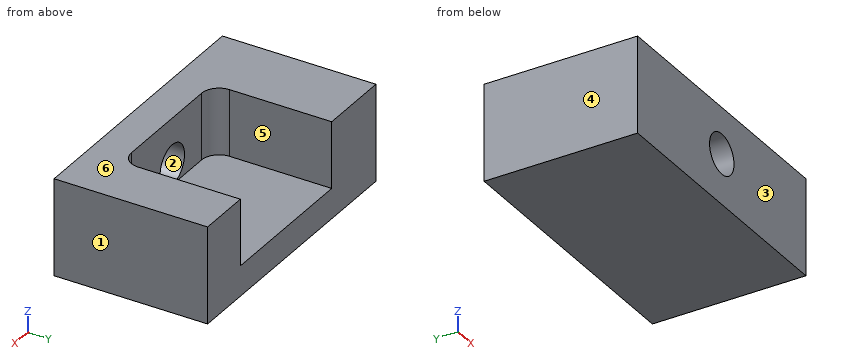
```python
from build123d import *

# Parameters (mm, degrees)
F0_W     = 56.4152672887
F0_H     = 35.5571135879
F1_DEPTH = 101.6
F3_DEPTH = 24.4419761002
F4_R     = 7.3661777125
F5_DEPTH = 25.4


with BuildPart() as f1:
    # F0 (on Right) → F1 (new body)
    with BuildSketch(Plane.YZ):
        with Locations((28.2076336443, 17.7785567939)):
            Rectangle(F0_W, F0_H)
    extrude(amount=F1_DEPTH)

    # F2 (on face) → F3 (cut)
    with BuildSketch(Plane.XY.offset(35.5571135879)):
        with BuildLine():
            Line((81.8312615156, 18.8686089426), (81.8312615156, 56.4152672887))
            Line((81.8312615156, 56.4152672887), (26.6845934093, 56.4152672887))
            Line((26.6845934093, 56.4152672887), (26.6845934093, 18.8686089426))
            ThreePointArc((26.6845934093, 18.8686089426), (28.5444653488, 14.3784808821), (33.0345934093, 12.5186089426))
            Line((33.0345934093, 12.5186089426), (75.4812615156, 12.5186089426))
            ThreePointArc((75.4812615156, 12.5186089426), (79.9713895762, 14.3784808821), (81.8312615156, 18.8686089426))
        make_face()
    extrude(amount=-F3_DEPTH, mode=Mode.SUBTRACT)

    # F4 (on face) → F5 (cut)
    with BuildSketch(Plane.XZ):
        with Locations((50.8, 18.4632241726)):
            Circle(F4_R)
    extrude(amount=-F5_DEPTH, mode=Mode.SUBTRACT)


solid = f1.part
```
Source: CAD feature listing. Evaluate the final solid. Frame: model axes, mm. Face numbers are marked on the shaded views. A direction names the side the tool comes from. Give positions to 0.01 mm unless a question says otherwise; leave off trailing zeros. Loops run counter-clockwise (first coordinate to the right, second up) from the corner with the lowest first, then second, coordinate; pieces in that order, holes last. Notation, with made-up numbers: (85.25, 27) - (103.25, 27) arc R17 ccw to (103.25, 32) - close; hole circle Ø9 at (49, 84.25). An arc over 180 degrees is marked (long way). Use CSV: the item, a comma, the result in double quotes. Start each with the question number.
1. Draft query along X for the marked faces 1, 2, 3 and 4. Return one class per face: +X half, -X half, draft (parallel to the pull), parting line (faces both ways), or undercut.
2. Reachability of the marked faces 5 and 6 from +Z, -Z, +X, -X, +Y, -Y: full face, straight path, thin tool, end or side. Return the list, or none.
3. Section A-A (y = 27). Output: boundary loops of the cut face in (x, z).
4. Section D-D (y = 6). Output: boundary loops of the cut face in (x, z).
5. Section C-C (z = 27). Output: boundary loops of the cut face in (x, y).
6. Section B-B (z = 19.5). Output: boundary loops of the cut face in (x, y), then the cut area to 3 significant figures.
7. Pin query (flat end, axial travel): pin 1 (22 mm diameter, centred on x = 43, y = 25.5, fed in from +Z); pin 2 (12 mm diameter, centred on x = 38.5, z = 19, fed in from +Y); pin 3 (12 mm diameter, centred on x = 70.5, z = 20.5, fed in from +Y). Return the tip coordinate at first contact, or that it passes through.
8. Ray query, L1, parallel to X at y = 26, z = 29.5; L2, parallel to Z at x = 50.8, y = 9.5; L3, parallel to Z at x = 50, y = 18. Return the intervals inside material, ascending.
Response:
1,face 1,"+X half"
1,face 2,"undercut"
1,face 3,"draft"
1,face 4,"-X half"
2,face 5,"+Z, +Y"
2,face 6,"+Z, +X, -X, +Y, -Y"
3,outline,"(0, 0) - (101.6, 0) - (101.6, 35.56) - (81.83, 35.56) - (81.83, 11.12) - (26.68, 11.12) - (26.68, 35.56) - (0, 35.56) - close"
4,outline,"(0, 0) - (101.6, 0) - (101.6, 35.56) - (0, 35.56) - close; hole circle Ø14.73 at (50.8, 18.46)"
5,outline,"(0, 0) - (101.6, 0) - (101.6, 56.42) - (81.83, 56.42) - (81.83, 18.87) arc R6.35 cw to (75.48, 12.52) - (33.03, 12.52) arc R6.35 cw to (26.68, 18.87) - (26.68, 56.42) - (0, 56.42) - close"
6,outline,"(0, 0) - (43.51, 0) - (43.51, 12.52) - (33.03, 12.52) arc R6.35 cw to (26.68, 18.87) - (26.68, 56.42) - (0, 56.42) - close; (58.09, 0) - (101.6, 0) - (101.6, 56.42) - (81.83, 56.42) - (81.83, 18.87) arc R6.35 cw to (75.48, 12.52) - (58.09, 12.52) - close"
6,area,"3,150 mm²"
7,pin 1,"z = 11.12"
7,pin 2,"y = 12.54"
7,pin 3,"y = 12.6"
8,L1,"0 to 26.68, 81.83 to 101.6"
8,L2,"0 to 11.1, 25.83 to 35.56"
8,L3,"0 to 11.12"
